Input: part model. Units: mm. Frame: model coordinates. A direction names the side the tool comes from. Round coordinates to 2 decimals unless told otherwise and drop trailing zeros. Write each loop counter-clockwise with the first axis right and the second up, starting at its lowest first coordinate (ties: lowest second). Pieces come first, ordered by that corner, then holes. Notation, with made-up numbers: (34.5, -11) -> (86.5, -11) arc R15 cw to (86.5, -6) -> close; hole circle Ø8 at (52, -6). An arc over 180 degrees is marked (long way). Use CSV: the item, a comma, the result in double quotes.
```python
from build123d import *

# Parameters (mm, degrees)
SKETCH1_R           = 6.35
BOSS_EXTRUDE1_DEPTH = 25.4
SKETCH2_R           = 7.9375
CUT_EXTRUDE1_DEPTH  = 26.4
FILLET1_R           = 3.175
CUT_EXTRUDE2_START  = -76.2
SKETCH3_R           = 2.5796875
CUT_EXTRUDE2_DEPTH  = 76.2
SKETCH4_R           = 1.35255
CUT_EXTRUDE3_DEPTH  = 15.748
SKETCH5_R           = 4.7625
CUT_EXTRUDE4_DEPTH  = 10.3886
SKETCH6_R           = 1.143
CUT_EXTRUDE5_DEPTH  = 6.35


with BuildPart() as part:
    # Sketch1 → Boss-Extrude1 (new body)
    with BuildSketch(Plane.XY):
        with BuildLine():
            Line((38.1, -34.925), (12.827, -34.925))
            Line((12.827, -34.925), (12.827, -13.92549629))
            ThreePointArc((12.827, -13.92549629), (13.023080834, -9.074919166), (8.17250371, -9.271))
            Line((8.17250371, -9.271), (-8.17250371, -9.271))
            ThreePointArc((-8.17250371, -9.271), (-13.023080834, -9.074919166), (-12.827, -13.92549629))
            Line((-12.827, -13.92549629), (-12.827, -34.925))
            Line((-12.827, -34.925), (-38.1, -34.925))
            Line((-38.1, -34.925), (-38.1, 34.925))
            Line((-38.1, 34.925), (28.575, 34.925))
            Line((28.575, 34.925), (28.575, 30.099))
            Line((28.575, 30.099), (28.575, 9.525))
            Line((28.575, 9.525), (38.1, 9.525))
            Line((38.1, 9.525), (38.1, -34.925))
        make_face()
        with Locations((0, 7.493)):
            Circle(SKETCH1_R, mode=Mode.SUBTRACT)
    extrude(amount=BOSS_EXTRUDE1_DEPTH)

    # Sketch2 → Cut-Extrude1 (cut, through all)
    with BuildSketch(Plane(origin=(0, 0, 0), x_dir=(-1, 0, 0), z_dir=(0, 0, -1))):
        with Locations((0, 7.493)):
            Circle(SKETCH2_R)
    extrude(amount=-CUT_EXTRUDE1_DEPTH, mode=Mode.SUBTRACT)

    # Fillet1
    fillet1_edges = [part.edges().sort_by_distance(p)[0] for p in [
        (-38.1, 34.925, 12.7),
        (28.575, 34.925, 12.7),
        (38.1, 9.525, 12.7),
    ]]
    fillet(fillet1_edges, radius=FILLET1_R)

    # Sketch3 → Cut-Extrude2 (cut)
    with BuildSketch(Plane(origin=(38.1, 0, 0), x_dir=(0, 0, -1), z_dir=(1, 0, 0)).offset(CUT_EXTRUDE2_START)):
        with Locations((-12.7, -22.225)):
            Circle(SKETCH3_R)
    extrude(amount=CUT_EXTRUDE2_DEPTH, mode=Mode.SUBTRACT)

    # Sketch4 → Cut-Extrude3 (cut)
    with BuildSketch(Plane.ZY.offset(38.1)):
        with Locations((12.7, 28.575)):
            Circle(SKETCH4_R)
    extrude(amount=-CUT_EXTRUDE3_DEPTH, mode=Mode.SUBTRACT)

    # Sketch5 → Cut-Extrude4 (cut)
    with BuildSketch(Plane(origin=(38.1, 0, 0), x_dir=(0, 0, -1), z_dir=(1, 0, 0))):
        with Locations((-12.7, -22.225)):
            Circle(SKETCH5_R)
    cut_extrude4 = extrude(amount=-CUT_EXTRUDE4_DEPTH, mode=Mode.SUBTRACT)

    # Mirror1: Cut-Extrude4 across plane
    add(cut_extrude4.mirror(Plane(origin=(0, 0, 0), x_dir=(0, 0, 1), z_dir=(1, 0, 0))), mode=Mode.SUBTRACT)

    # Sketch6 → Cut-Extrude5 (cut)
    with BuildSketch(Plane(origin=(28.575, 0, 0), x_dir=(0, 0, -1), z_dir=(1, 0, 0))):
        with Locations((-7.62, 14.859)):
            Circle(SKETCH6_R)
        with Locations((-7.62, 24.765)):
            Circle(SKETCH6_R)
    extrude(amount=-CUT_EXTRUDE5_DEPTH, mode=Mode.SUBTRACT)


solid = part.part
```
Item 1: Section query C-C on z = 12.7. Give the number of separate pieces and of enclosed holes in the cut face, plus the area to 3 significant figures.
Worked answers:
separate pieces,"3"
enclosed holes,"1"
area,"3,810 mm²"
Item 2: First-contact query: pin 1 Ø5 at (y, z) = (17, 20.5) entering from +X (3 decimals); pin 2 Ø13 at (x, z) = (-1.5, 15.5) entering from -Y; pin 3 Ø3 at (y, z) = (-22.225, 12.7) entering from +X; pin 4 Ø0.7 at (y, z) = (24.5, 8) entering from +X (3 decimals). Flat tips, straight axial feed; report the tip coordinate or a pass-through.
Worked answers:
pin 1,"stops at x = 28.575"
pin 2,"stops at y = -9.27"
pin 3,"passes through"
pin 4,"stops at x = 22.225"
Item 3: Pull-direction query (Y, two-part tool) for faces 1 (the face through (1.033, 15.363, 12.522)), 2 (the face through (-25, -34.925, 13)), 3 (the face through (27.67, 33.97, 12.88)); classes: +Y half, -Y half, draft (parallel to the pull), parting line (faces both ways), or undercut.
Worked answers:
face 1,"undercut"
face 2,"-Y half"
face 3,"+Y half"
Item 4: Section query A-A on y = -28. Return the cut outline in (x, z), plus the area to 3 significant figures.
Worked answers:
outline,"(-38.1, 0) -> (-12.83, 0) -> (-12.83, 25.4) -> (-38.1, 25.4) -> close; (12.83, 0) -> (38.1, 0) -> (38.1, 25.4) -> (12.83, 25.4) -> close"
area,"1,280 mm²"
Item 5: Section query D-D on x = -30. Return the cut outline in (y, z) (1 decimal).
Worked answers:
outline,"(-34.9, 0) -> (34.9, 0) -> (34.9, 25.4) -> (-34.9, 25.4) -> close; hole circle Ø9.5 at (-22.2, 12.7); hole circle Ø2.7 at (28.6, 12.7)"
Item 6: Section query B-B on x = 0. Return the cut outline in (y, z) (1 decimal).
Worked answers:
outline,"(-9.3, 0) -> (-0.4, 0) -> (-0.4, 25.4) -> (-9.3, 25.4) -> close; (15.4, 0) -> (34.9, 0) -> (34.9, 25.4) -> (15.4, 25.4) -> close"
Item 7: Line query: line 1 (Y direction, x = -32.25, z = 12.7) (1 decimal); line 2 (X direction, y = -14, z = 15.25); line 3 (X direction, y = -11.5, z = 7). Output: solid intervals per line, ascending.
Worked answers:
line 1,"y = -34.9 to -27, -17.5 to 27.2, 29.9 to 34.9"
line 2,"x = -38.1 to -12.83, 12.83 to 38.1"
line 3,"x = -38.1 to -13.99, 13.99 to 38.1"
Item 8: Set-up query: faces 4 (the face through (32.98, -18.21, 10.14)), 5 (the face through (-30.336, 27.255, 12.407)), 6 (the face through (28.575, 21, 13)). Return all of +Z, -Z, +X, -X, +Y, -Y with unobstructed straight access to the full face (end or side cutting, diameter ignored); none if empty.
Worked answers:
face 4,"+X"
face 5,"-X"
face 6,"+Z, -Z, +X, +Y"
